For this review, use the dimensioned drawing (mm, ordinates from the lowest corner) and the shaded views. Coordinates: 2 decimals unless noted, no trailing zeros. Loops run counter-clockwise (first coordinate to the right, second up) from the corner with the lowest first, then second, coordinate; pieces in that order, holes last. Notation, with made-up numbers: (85.5, 28.25) - (100.5, 28.25) arc R26 ccw to (100.5, 59.25) - close; hole circle Ø2 at (70, 18). An arc over 180 degrees is marked (long way). Answer in a Markdown table with one row per item. Add a question column.
(1) We need section A-A on x = 59.5. Write out the cut boundary in (y, z).
(2) We need section B-B on z = 6.75. Write out the cut boundary in (x, y).
(3) We need section C-C on y = 6.35. Write out the cut boundary in (x, z).
(4) For line 1 along X through (y, z) = (6.35, 4); line 2 along Y through (x, z) = (59.5, 9.5); line 3 along X through (y, z) = (5.5, 10.75), list the stretches that pass through material, from the lowest coordinate up.
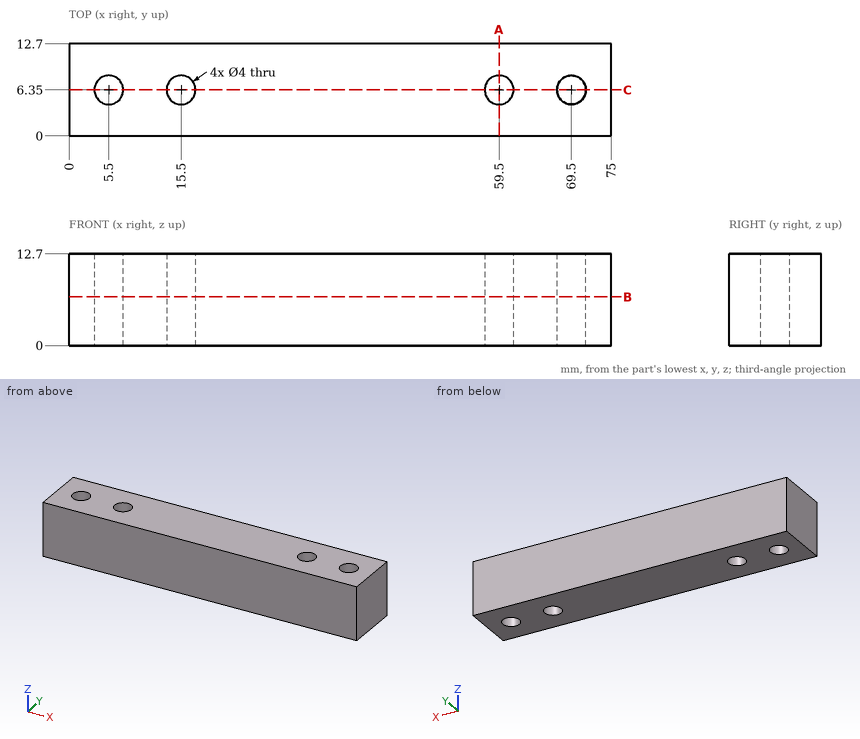
Outcome:
| question | item | result |
|---|---|---|
| 1 | outline | (0, 0) - (4.35, 0) - (4.35, 12.7) - (0, 12.7) - close; (8.35, 0) - (12.7, 0) - (12.7, 12.7) - (8.35, 12.7) - close |
| 2 | outline | (0, 0) - (75, 0) - (75, 12.7) - (0, 12.7) - close; hole circle Ø4 at (5.5, 6.35); hole circle Ø4 at (15.5, 6.35); hole circle Ø4 at (59.5, 6.35); hole circle Ø4 at (69.5, 6.35) |
| 3 | outline | (0, 0) - (3.5, 0) - (3.5, 12.7) - (0, 12.7) - close; (7.5, 0) - (13.5, 0) - (13.5, 12.7) - (7.5, 12.7) - close; (17.5, 0) - (57.5, 0) - (57.5, 12.7) - (17.5, 12.7) - close; (61.5, 0) - (67.5, 0) - (67.5, 12.7) - (61.5, 12.7) - close; (71.5, 0) - (75, 0) - (75, 12.7) - (71.5, 12.7) - close |
| 4 | line 1 | 0 to 3.5, 7.5 to 13.5, 17.5 to 57.5, 61.5 to 67.5, 71.5 to 75 |
| 4 | line 2 | 0 to 4.35, 8.35 to 12.7 |
| 4 | line 3 | 0 to 3.69, 7.31 to 13.69, 17.31 to 57.69, 61.31 to 67.69, 71.31 to 75 |
